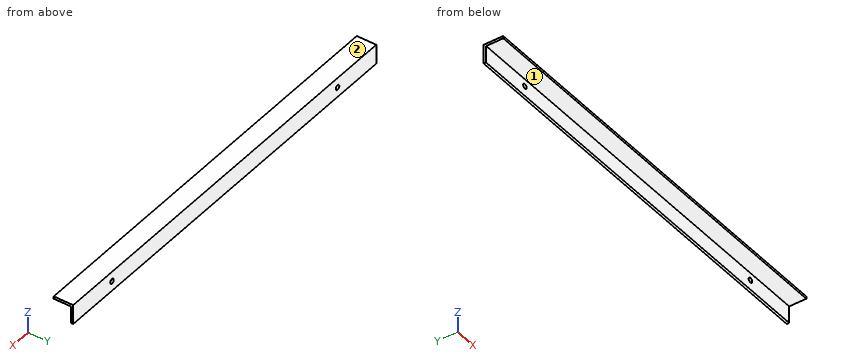
Autodesk Inventor part; units mm, degrees
ref_plane "YZ Plane" through (0, 0, 0) normal (1, 0, 0) x (0, 1, 0)
ref_plane "XZ Plane" through (0, 0, 0) normal (0, 1, 0) x (-1, 0, 0)
ref_plane "XY Plane" through (0, 0, 0) normal (0, 0, 1) x (1, 0, 0)
sketch "Sketch1" plane through (0, 0, 0) normal (1, 0, 0) x (0, 1, 0)
  line L0 (0, 0) -> (-3.175, 0)
  line L1 (-3.175, 0) -> (-3.175, -25.4)
  line L2 (-3.175, -25.4) -> (0, -25.4)
  line L3 (0, -25.4) -> (0, 0)
  line L4 (0, 0) -> (-25.4, 0)
  line L5 (-25.4, 0) -> (-25.4, -3.175)
  line L6 (-25.4, -3.175) -> (0, -3.175)
  line L7 (0, -3.175) -> (0, 0)
  dimension "d0" = 3.175
  dimension "d1" = 25.4
  dimension "d2" = 25.4
  dimension "d3" = 3.175
extrude "Extrusion1" add sketch "Sketch1" along normal blind 546.1
sketch "Sketch2" plane through (0, 0, 0) normal (0, 1, 0) x (1, 0, 0)
  line L0 (0, 25.4) -> (0, 0)
  line L1 (0, 0) -> (546.1, 0)
  line L2 (546.1, 25.4) -> (546.1, 0)
  point P0 (476.25, 12.7)
  point P1 (69.85, 12.7)
  dimension "d6" = 69.85
  dimension "d7" = 12.7
  dimension "d8" = 69.85
  dimension "d9" = 12.7
hole "Hole1" at (476.25, 0, -12.7) at (69.85, 0, -12.7) direction (0, -1, 0) diameter 6.35 end through all
properties part number "pool noodle guard 1x1 angle"
Check sheet for the modelled part. Datum: model origin and axes. Units: mm. Face numbers are marked on the shaded views. A direction names the side the tool comes from. Coordinates: 2 decimals unless noted, no trailing zeros. Order: outer loops, then holes, each group sorted by start corner. A loop starts at its lowest first (then second) coordinate and runs counter-clockwise, first axis right, second up. Notation, with made-up numbers: M 22.5,10 L 53.5,10 A24 ccw 53.5,39 Z; hole C 2,37.5 d11. An arc over 180 degrees is marked long. Write each question's results on one line, items separated by ' | '. Start each with the question number.
1. Cross-section at A-A on x = 153.5. Record the cut outline in (y, z) (3 decimals).
2. Material ranges on probe 1 along X at (y, z) = (-1, -12.7) (3 decimals); probe 2 along Z at (x, y) = (69.85, -1.5) (3 decimals); probe 3 along Z at (x, y) = (510.5, -13.5) (3 decimals), recorded low to high.
3. Go/stop test with flat-tipped pins: P1, Ø6.5, axis at x = 211.5, y = -10, coming from the -Z side (3 decimals); P2, Ø8.5, axis at x = 69.85, z = -12.7, coming from the -Y side (3 decimals). Record where each tip stops, or that it passes through.
4. Cross-section at B-B on y = -11. Record the cut outline in (x, z) (3 decimals).
5. Access from +Z, -Z, +X, -X, +Y, -Y to the whole of each face (thin tool, end or side, straight path). Record for the marked faces 1 and 2.
Checks:
1) outline: M -25.4,-3.175 L -3.175,-3.175 L -3.175,-25.4 L 0,-25.4 L 0,0 L -25.4,0 Z
2) probe 1: x = 0 to 66.675, 73.025 to 473.075, 479.425 to 546.1 | probe 2: z = -25.4 to -15.875, -9.525 to 0 | probe 3: z = -3.175 to 0
3) P1: stops at z = -3.175 | P2: stops at y = -3.175
4) outline: M 0,-3.175 L 546.1,-3.175 L 546.1,0 L 0,0 Z
5) face 1: -Z, +X, -X, -Y | face 2: +Z, +X, -X, +Y, -Y
